The model under review builds one solid part; all positions refer to its coordinate system, in mm. Face numbers are marked on the shaded views. Give positions to 0.01 mm unless a question says otherwise; leave off trailing zeros. Loops run counter-clockwise (first coordinate to the right, second up) from the corner with the lowest first, then second, coordinate; pieces in that order, holes last. Notation, with made-up numbers: (1.25, -25) - (12.25, -25) arc R26 cw to (12.25, 4) - close; hole circle Ø11 at (68.25, 17). An arc over 180 degrees is marked (long way). Return JSON: item names as keys, results as strings. Group by question number.
Autodesk Inventor part; units mm, degrees
ref_plane "YZ Plane" through (0, 0, 0) normal (1, 0, 0) x (0, 1, 0)
ref_plane "XZ Plane" through (0, 0, 0) normal (0, 1, 0) x (-1, 0, 0)
ref_plane "XY Plane" through (0, 0, 0) normal (0, 0, 1) x (1, 0, 0)
sketch "スケッチ1" plane through (0, 0, 0) normal (0, 0, 1) x (1, 0, 0)
  circle A0 centre (0, 0) radius 18
  dimension "d0" = 36
extrude "押し出し1" add sketch "スケッチ1" along normal blind 3.25
sketch "スケッチ2" plane through (0, 0, 3.25) normal (0, 0, 1) x (1, 0, 0)
  circle A0 centre (0, 0) radius 6
  point P0 (0, 6)
  point P1 (-6, 0)
  point P2 (0, -6)
  point P3 (6, 0)
  dimension "d3" = 12
  dimension "d6" = 360
hole "穴1" at (0, 6, 3.25) at (-6, 0, 3.25) at (0, -6, 3.25) at (6, 0, 3.25) direction (0, 0, -1) diameter 3.2 end through all counterbore diameter 6.5 counterbore depth 4
sketch "スケッチ3" plane through (0, 0, 0) normal (0, 0, -1) x (-1, 0, 0)
  circle A0 centre (0, 0) radius 8.5
  point P0 (-6.0104, 6.0104)
  point P1 (-6.0104, -6.0104)
  point P2 (6.0104, -6.0104)
  point P3 (6.0104, 6.0104)
  dimension "d15" = 17
  dimension "d18" = 360
hole "穴2" at (6.0104, 6.0104, 0) at (6.0104, -6.0104, 0) at (-6.0104, -6.0104, 0) at (-6.0104, 6.0104, 0) direction (0, 0, 1) diameter 3.2 end through all
sketch "スケッチ4" plane through (0, 0, 0) normal (0, 0, -1) x (-1, 0, 0)
  circle A0 centre (0, 0) radius 3.25
  dimension "d27" = 6.5
extrude "押し出し2" cut sketch "スケッチ4" against normal blind 8
fillet "フィレット1" radius 0.5 8 edges at (-1.25, -3, 1.625) (1.25, -3, 1.625) (3, -1.25, 1.625) (3, 1.25, 1.625) (1.25, 3, 1.625) (-1.25, 3, 1.625) (-3, 1.25, 1.625) (-3, -1.25, 1.625)
sketch "スケッチ5" plane through (0, 0, 3.25) normal (0, 0, 1) x (1, 0, 0)
  circle A0 centre (0, 0) radius 15
  point P0 (0, -15)
  point P1 (10.6066, -10.6066)
  point P2 (15, 0)
  point P3 (10.6066, 10.6066)
  point P4 (0, 15)
  point P5 (-10.6066, 10.6066)
  point P6 (-15, 0)
  point P7 (-10.6066, -10.6066)
  dimension "d31" = 30
  dimension "d34" = 360
hole "穴3" at (0, -15, 3.25) at (10.6066, -10.6066, 3.25) at (15, 0, 3.25) at (10.6066, 10.6066, 3.25) at (0, 15, 3.25) at (-10.6066, 10.6066, 3.25) at (-15, 0, 3.25) at (-10.6066, -10.6066, 3.25) direction (0, 0, -1) diameter 3.2 end through all
properties part number "s_base5"
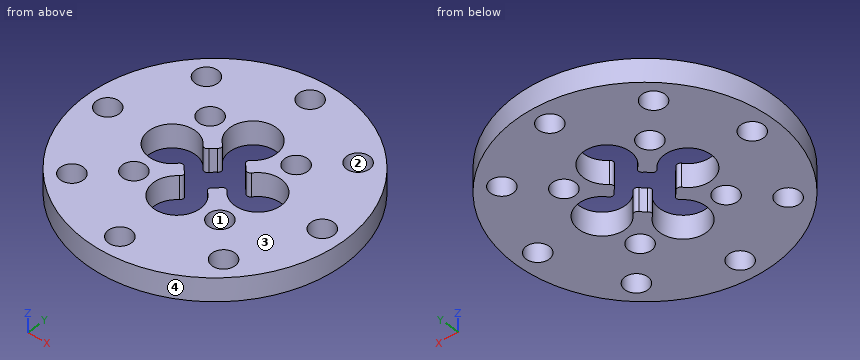
1) We need section B-B, the plane y = -15. Write out the cut boundary in (x, z), plus the area to 3 significant figures.
2) For pin 1 Ø1 at (y, z) = (3.5, 2.5) entering from -X; pin 2 Ø1 at (y, z) = (-2, 2.5) entering from +X, all flat-tipped, find the tip position at first contact; note any pin that passes through.
3) We need section A-A, the plane x = 0. Write out the cut boundary in (y, z), plus the area to 3 significant figures.
4) To check wall thickness, follow line 1 (Y direction, x = -2.5, z = 2.65); line 2 (Y direction, x = 0, z = 1.4); line 3 (X direction, y = 6, z = 2.65). State the ranges of each line that lie inside material, in increasing order.
5) We need section D-D, the plane y = -7. Write out the cut boundary in (x, z).
6) Draft analysis for pull direction X (two halves, no side actions). For the marked faces 1, 2, 3 and 4, state which applies: +X half, -X half, draft (parallel to the pull), parting line (faces both ways), or undercut.
Findings:
{
 "1": {"outline": "(-9.95, 0) - (-1.6, 0) - (-1.6, 3.25) - (-9.95, 3.25) - close; (1.6, 0) - (9.95, 0) - (9.95, 3.25) - (1.6, 3.25) - close", "area": "54.3 mm^2"},
 "2": {"pin 1": "stops at x = -17.75", "pin 2": "stops at x = 17.94"},
 "3": {"outline": "(-18, 0) - (-16.6, 0) - (-16.6, 3.25) - (-18, 3.25) - close; (-13.4, 0) - (-9.25, 0) - (-9.25, 3.25) - (-13.4, 3.25) - close; (9.25, 0) - (13.4, 0) - (13.4, 3.25) - (9.25, 3.25) - close; (16.6, 0) - (18, 0) - (18, 3.25) - (16.6, 3.25) - close", "area": "36.1 mm^2"},
 "4": {"line 1": "y = -17.83 to -8.08, -3.92 to -2.08, 2.08 to 3.92, 8.08 to 17.83", "line 2": "y = -18 to -16.6, -13.4 to -9.25, 9.25 to 13.4, 16.6 to 18", "line 3": "x = -16.97 to -7.61, -4.41 to -3.25, 3.25 to 4.41, 7.61 to 16.97"},
 "5": {"outline": "(-16.58, 0) - (-7.27, 0) - (-7.27, 3.25) - (-16.58, 3.25) - close; (-4.75, 0) - (-3.09, 0) - (-3.09, 3.25) - (-4.75, 3.25) - close; (3.09, 0) - (4.75, 0) - (4.75, 3.25) - (3.09, 3.25) - close; (7.27, 0) - (16.58, 0) - (16.58, 3.25) - (7.27, 3.25) - close"},
 "6": {"face 1": "undercut", "face 2": "undercut", "face 3": "draft", "face 4": "parting line"}
}
